from build123d import *

# Parameters (mm, degrees)
SKETCH1_R                = 29
BOSS_EXTRUDE1_DEPTH      = 13
BOSS_EXTRUDE1_DEPTH_BACK = 13
SKETCH2_R                = 7
CUT_EXTRUDE1_DEPTH       = 1.5


with BuildPart() as part:
    # Sketch1 → Boss-Extrude1 (new body, two sides)
    with BuildSketch(Plane.XY) as boss_extrude1_sk:
        Circle(SKETCH1_R)
        with BuildLine():
            Line((-5.95294045, 0.75), (-6.45294045, 0.75))
            Line((-6.45294045, 0.75), (-6.45294045, -0.75))
            Line((-6.45294045, -0.75), (-5.95294045, -0.75))
            ThreePointArc((-5.95294045, -0.75), (6, 0), (-5.95294045, 0.75))
        make_face(mode=Mode.SUBTRACT)
    extrude(amount=BOSS_EXTRUDE1_DEPTH)
    extrude(boss_extrude1_sk.sketch, amount=-BOSS_EXTRUDE1_DEPTH_BACK)

    # Sketch2 → Cut-Extrude1 (cut)
    with BuildSketch(Plane.XY.offset(13)):
        Circle(SKETCH2_R)
    cut_extrude1 = extrude(amount=-CUT_EXTRUDE1_DEPTH, mode=Mode.SUBTRACT)

    # Mirror1: Cut-Extrude1 across plane
    add(cut_extrude1.mirror(Plane.XY), mode=Mode.SUBTRACT)


solid = part.part
Can you work these out from the model? Positions are in its coordinate system, mm. A direction names the side the tool comes from. Coordinates: 2 decimals unless noted, no trailing zeros. Write each loop counter-clockwise with the first axis right and the second up, starting at its lowest first coordinate (ties: lowest second). Pieces come first, ordered by that corner, then holes. Notation, with made-up numbers: (-34.75, -28) -> (-24.75, -28) arc R14 ccw to (-24.75, -10) -> close; hole circle Ø2 at (82.25, 69). An arc over 180 degrees is marked (long way). Write each question's results on one line, items separated by ' | '. Start each with the question number.
Q1. Imagine slicing it at A-A (x = 0). Write out the boundary of the cut face in (y, z), then the cut area to 3 significant figures.
Q2. Imagine slicing it at C-C (z = 6.25). Write out the boundary of the cut face in (x, y).
Q3. Imagine slicing it at B-B (y = 0). Write out the boundary of the cut face in (x, z).
Q4. Imagine slicing it at D-D (x = -21). Write out the boundary of the cut face in (y, z).
Q5. I'm going to push flat-ended pins straight in: pin 1 (19 mm diameter, centred on x = 0, y = 0, fed in from -Z); pin 2 (1 mm diameter, centred on y = -21, z = 8, fed in from +X); pin 3 (4 mm diameter, centred on x = -1, z = 2.5, fed in from -Y); pin 4 (5 mm diameter, centred on x = -21.5, z = -10.5, fed in from +Y). Where does each tip first touch, or does it pass through?
Q6. If I drill on probe 1 along Y at (x, z) = (0, 12.05); probe 2 along Y at (x, z) = (0, 6.25); probe 3 along Y at (x, z) = (-14, -8), over which ranges is the centre line in solid material (lowest first)?
Q7. We'd pull the mould along X, two halves only. Please class faces 4 (the face through (13.38, -25.73, 0.18)), 5 (the face through (2, -6, 11.5)), 6 (the face through (6, -6, 13)): +X half, -X half, draft (parallel to the pull), parting line (faces both ways), or undercut.
Q8. On a 3-axis mill with a long thin cutter (end or side, diameter ignored), from which of +Z, -Z, +X, -X, +Y, -Y can I reach the whole of each face in a straight line? I mean faces 1 (the face through (6.466, -2.681, 12.26)), 2 (the face through (-6.453, 0, 0)), 3 (the face through (2, -6, -11.5)). Say none if no direction works.
Taken from the geometry:
1) outline: (-29, -13) -> (-7, -13) -> (-7, -11.5) -> (-6, -11.5) -> (-6, 11.5) -> (-7, 11.5) -> (-7, 13) -> (-29, 13) -> close; (6, -11.5) -> (7, -11.5) -> (7, -13) -> (29, -13) -> (29, 13) -> (7, 13) -> (7, 11.5) -> (6, 11.5) -> close | area: 1,190 mm^2
2) outline: circle Ø58 at (0, 0); hole (-6.45, -0.75) -> (-5.95, -0.75) arc R6 ccw (long way) to (-5.95, 0.75) -> (-6.45, 0.75) -> close
3) outline: (-29, -13) -> (-7, -13) -> (-7, -11.5) -> (-6.45, -11.5) -> (-6.45, 11.5) -> (-7, 11.5) -> (-7, 13) -> (-29, 13) -> close; (6, -11.5) -> (7, -11.5) -> (7, -13) -> (29, -13) -> (29, 13) -> (7, 13) -> (7, 11.5) -> (6, 11.5) -> close
4) outline: (-20, -13) -> (20, -13) -> (20, 13) -> (-20, 13) -> close
5) pin 1: stops at z = -13 | pin 2: stops at x = 20.51 | pin 3: stops at y = -29 | pin 4: stops at y = 21.91
6) probe 1: y = -29 to -7, 7 to 29 | probe 2: y = -29 to -6, 6 to 29 | probe 3: y = -25.4 to 25.4
7) face 4: parting line | face 5: undercut | face 6: draft
8) face 1: +Z | face 2: +Z, -Z | face 3: -Z
